Part model, mm, in its own coordinate system. Round coordinates to 2 decimals unless told otherwise and drop trailing zeros. Order: outer loops, then holes, each group sorted by start corner. A loop starts at its lowest first (then second) coordinate and runs counter-clockwise, first axis right, second up. Notation, with made-up numbers: M 72.5,-22 L 100.5,-22 A20 ccw 100.5,2 Z; hole C 88,86.25 d11. An arc over 180 degrees is marked long. One line per question, with ' | ' between items.
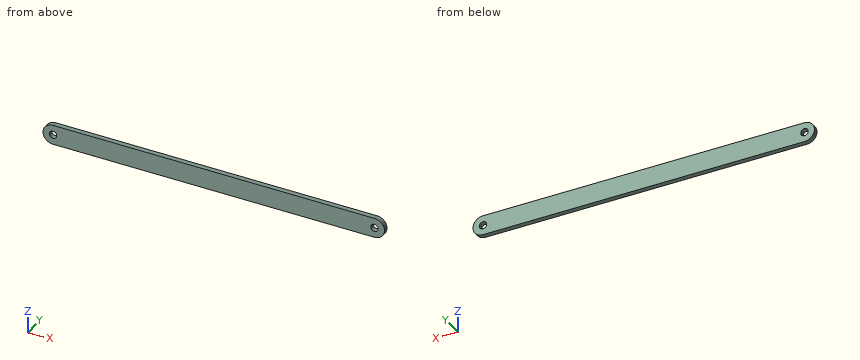
Autodesk Inventor part; units mm, degrees
ref_plane "YZ Plane" through (0, 0, 0) normal (1, 0, 0) x (0, 1, 0)
ref_plane "XZ Plane" through (0, 0, 0) normal (0, 1, 0) x (-1, 0, 0)
ref_plane "XY Plane" through (0, 0, 0) normal (0, 0, 1) x (1, 0, 0)
sketch "Sketch1" plane through (0, 0, 0) normal (0, 1, 0) x (-1, 0, 0)
  circle A0 centre (102.6747, -1.4203) radius 2.1844 construction
  circle A1 centre (-100.5253, -1.4203) radius 2.1844 construction
  circle A2 centre (102.6747, -1.4203) radius 2.3495
  circle A3 centre (-100.5253, -1.4203) radius 2.3495
  circle A4 centre (102.6747, -1.4203) radius 6.35
  circle A5 centre (-100.5253, -1.4203) radius 6.35
  line L0 (102.6747, -7.7703) -> (-100.5253, -7.7703)
  line L1 (102.6747, 4.9297) -> (-100.5253, 4.9297)
  point P0 (0, 0)
  dimension "d0" = 4.699
  dimension "d1" = 4.699
  dimension "d2" = 12.7
  dimension "d3" = 12.7
extrude "Plate1" add sketch "Sketch1" along normal blind 3.048
equation "\"d4\" = Thickness"
equation "\"BendRadius\" = Thickness"
equation "\"BendReliefWidth\" = Thickness"
equation "\"BendReliefDepth\" = 0.5 * Thickness"
equation "\"CornerReliefSize\" = 4 * Thickness"
equation "\"MinimumRemnant\" = 2 * Thickness"
equation "\"TransitionRadius\" = BendRadius"
equation "\"JacobiRadiusSize\" = BendRadius"
equation "\"GapSize\" = Thickness"
properties part number "undersideStrip"
1) Drop flat-ended pins along their axis: pin 1 (1 mm diameter, centred on y = 0.5, z = -3.5, fed in from +X); pin 2 (7.5 mm diameter, centred on x = -102.67, z = -1.42, fed in from +Y). Give the stop position or say it passes through.
The answers:
pin 1: stops at x = 106.68 | pin 2: stops at y = 3.05
2) Saw through at A-A (y = 1.6). List the corners of the cut face in (x, z).
The answers:
outline: M -102.67,-7.77 L 100.53,-7.77 A6.35 ccw 100.53,4.93 L -102.67,4.93 A6.35 ccw Z; hole C -102.67,-1.42 d4.7; hole C 100.53,-1.42 d4.7
3) Probe line 1 (X direction, y = 0.15, z = -1); line 2 (X direction, y = 1.25, z = -1.25); line 3 (X direction, y = 0.6, z = -4.5). List the from-to ranges inside material, lowest first. Write a range as [from, to].
The answers:
line 1: x = [-109.01, -104.99], [-100.36, 98.21], [102.84, 106.86] | line 2: x = [-109.02, -105.02], [-100.33, 98.18], [102.87, 106.87] | line 3: x = [-108.23, 106.08]
